Part print with two shaded views. Sizes in mm from the minimum x, y, z corner. Give positions to 0.01 mm unless a question says otherwise; leave off trailing zeros. Order: outer loops, then holes, each group sorted by start corner. A loop starts at its lowest first (then second) coordinate and runs counter-clockwise, first axis right, second up. Notation, with made-up numbers: M -32.75,-12.75 L 4.25,-12.75 A9 cw 4.25,3.25 Z; hole C 35,86 d4. An arc over 180 degrees is marked long. Return JSON: item names as keys, results as strings.
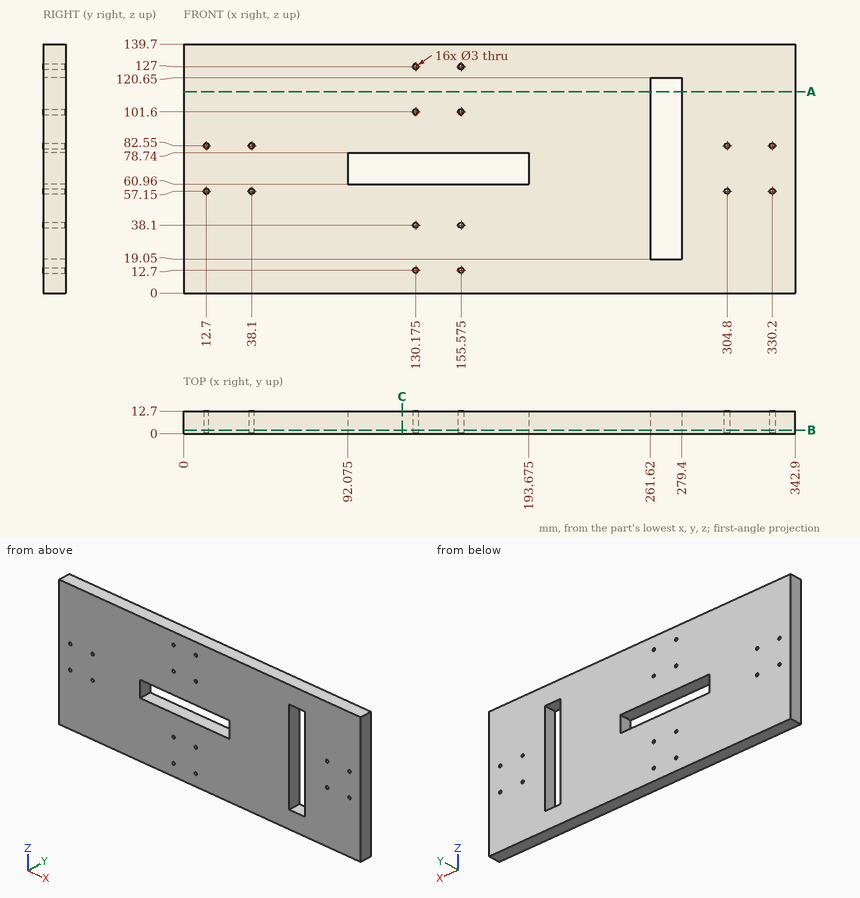
Q1. Probe line 1 along X through (y, z) = (7.25, 101.6) (3 decimals); line 2 along Z through (x, y) = (304.8, 9.25); line 3 along X through (y, z) = (4.5, 62.5) (3 decimals). List the from-to ranges inside material, lowest first.
Established:
{"line 1": "x = 0 to 128.675, 131.675 to 154.075, 157.075 to 261.62, 279.4 to 342.9", "line 2": "z = 0 to 55.65, 58.65 to 81.05, 84.05 to 139.7", "line 3": "x = 0 to 92.075, 193.675 to 261.62, 279.4 to 342.9"}
Q2. Band-saw the part on C-C (x = 122.5). Give the cut face in (y, z).
Established:
{"outline": "M 0,0 L 12.7,0 L 12.7,60.96 L 0,60.96 Z; M 0,78.74 L 12.7,78.74 L 12.7,139.7 L 0,139.7 Z"}
Q3. Band-saw the part on A-A (z = 113). Give the cut face in (x, y).
Established:
{"outline": "M 0,0 L 261.62,0 L 261.62,12.7 L 0,12.7 Z; M 279.4,0 L 342.9,0 L 342.9,12.7 L 279.4,12.7 Z"}
Q4. Pin check, flat tip, straight feed: pin 1 (2.5 mm diameter, centred on x = 304.8, z = 57.15, fed in from +Y). Stop position of the tip, or through.
Established:
{"pin 1": "passes through"}
Q5. Band-saw the part on B-B (y = 2). Give the number of separate pieces and of enclosed holes in the cut face, then the cut area to 3 significant figures.
Established:
{"separate pieces": "1", "enclosed holes": "18", "area": "44,200 mm²"}
